Verification items for the finished model (mm, model axes). A direction names the side the tool comes from. Give positions to 0.01 mm unless a question says otherwise; leave off trailing zeros. Write each loop counter-clockwise with the first axis right and the second up, starting at its lowest first coordinate (ties: lowest second). Pieces come first, ordered by that corner, then holes. Notation, with made-up numbers: (47.25, -13.5) - (97.25, -13.5) arc R6 cw to (97.25, -7.5) - close; hole circle Ø3 at (-25.75, 25.5). An arc over 180 degrees is marked (long way). Put each result on its own line as item: value.
from build123d import *

# Parameters (mm, degrees)
BOSS_EXTRUDE1_DEPTH      = 16.65
BOSS_EXTRUDE1_DEPTH_BACK = 16.65
CHAMFER1_SIZE            = 1.5
SKETCH2_R                = 1.75
BOSS_EXTRUDE2_DEPTH      = 1
SKETCH3_R                = 0.6
BOSS_EXTRUDE3_DEPTH      = 5
SKETCH4_W                = 29.3
SKETCH4_H                = 9.15
CUT_EXTRUDE1_DEPTH       = 5.5
CHAMFER2_SIZE            = 0.5


with BuildPart() as part:
    # Sketch1 → Boss-Extrude1 (new, two sides: drawn at the far end of the back side and taken through both)
    with BuildSketch(Plane(origin=(0, 0, 0), x_dir=(0, 0, -1), z_dir=(1, 0, 0)).offset(-BOSS_EXTRUDE1_DEPTH_BACK)):
        Polygon((-24.775, 15.2), (-8.275, 15.2), (-3.825, 10.75), (24.775, 10.75), (24.775, 0), (-16.575, 0), (-19.975, 3.4), (-24.775, 3.4), align=None)
    extrude(amount=BOSS_EXTRUDE1_DEPTH + BOSS_EXTRUDE1_DEPTH_BACK)

    # Chamfer1
    chamfer1_edges = [part.edges().sort_by_distance(p)[0] for p in [
        (-16.65, 1.7, 18.275),
        (-16.65, 0, -4.1),
        (0, 10.75, -24.775),
        (0, 0, -24.775),
        (-16.65, 5.375, -24.775),
        (-16.65, 10.75, -10.475),
        (-16.65, 12.975, 6.05),
        (16.65, 3.4, 22.375),
        (16.65, 1.7, 18.275),
        (16.65, 0, -4.1),
        (16.65, 5.375, -24.775),
        (16.65, 10.75, -10.475),
        (16.65, 12.975, 6.05),
        (16.65, 15.2, 16.525),
        (-16.65, 15.2, 16.525),
        (-16.65, 3.4, 22.375),
    ]]
    chamfer(chamfer1_edges, length=CHAMFER1_SIZE)

    # Sketch2 → Boss-Extrude2 (add)
    with BuildSketch(Plane(origin=(0, 0, -24.775), x_dir=(-1, 0, 0), z_dir=(0, 0, -1))):
        with Locations((-9.45, 6)):
            Circle(SKETCH2_R)
        with Locations((9.55, 6)):
            Circle(SKETCH2_R)
    extrude(amount=BOSS_EXTRUDE2_DEPTH)

    # Sketch3 → Boss-Extrude3 (add)
    with BuildSketch(Plane(origin=(0, 0, -25.775), x_dir=(-1, 0, 0), z_dir=(0, 0, -1))):
        with Locations((-9.45, 6)):
            Circle(SKETCH3_R)
        with Locations((9.55, 6)):
            Circle(SKETCH3_R)
    extrude(amount=BOSS_EXTRUDE3_DEPTH)

    # Sketch4 → Cut-Extrude1 (cut)
    with BuildSketch(Plane.XY.offset(24.775)):
        with Locations((0, 9.3)):
            Rectangle(SKETCH4_W, SKETCH4_H)
    extrude(amount=-CUT_EXTRUDE1_DEPTH, mode=Mode.SUBTRACT)

    # Chamfer2
    chamfer2_edges = [part.edges().sort_by_distance(p)[0] for p in [
        (-14.65, 9.3, 24.775),
        (0, 4.725, 24.775),
        (14.65, 9.3, 24.775),
        (0, 13.875, 24.775),
    ]]
    chamfer(chamfer2_edges, length=CHAMFER2_SIZE)


solid = part.part
Q1. Set-up check for faces 1 (the face through (0, 10.75, -10)), 2 (the face through (0, 13.875, 22)), 3 (the face through (0, 3.4, 22)), 4 (the face through (-9.17, 4.29, -25.27)): record each of +Z, -Z, +X, -X, +Y, -Y from which the full face is reachable in a straight line by a thin tool's end or side.
Answers follow:
face 1: -Z, +X, -X, +Y
face 2: +Z
face 3: +Z, +X, -X, -Y
face 4: -Z
Q2. Go/stop test with flat-tipped pins: pin 1 Ø2.5 at (x, y) = (-6, 3.5) entering from -Z (3 decimals); pin 2 Ø3 at (x, y) = (9, 5.5) entering from -Z (3 decimals); pin 3 Ø6 at (x, y) = (-12, 10) entering from -Z (3 decimals); pin 4 Ø1.5 at (x, z) = (7, 21) entering from -Y. Record where each tip stops, or that it passes through.
Answers follow:
pin 1: stops at z = -24.775
pin 2: stops at z = -30.775
pin 3: stops at z = -25.775
pin 4: stops at y = 3.4
Q3. Section check D-D, the plane x = 14. Record the cut outline in (y, z) (3 decimals), plus the area to 3 significant figures.
Answers follow:
outline: (0, -23.275) - (1.5, -24.775) - (9.25, -24.775) - (10.75, -23.275) - (10.75, 3.825) - (15.2, 8.275) - (15.2, 24.775) - (14.375, 24.775) - (13.875, 24.275) - (13.875, 19.275) - (4.725, 19.275) - (4.725, 24.275) - (4.225, 24.775) - (3.4, 24.775) - (3.4, 19.975) - (0, 16.575) - close
area: 541 mm2
Q4. Section check B-B, the plane y = 6. Record the cut outline in (x, z) (3 decimals), plus the area to 3 significant figures.
Answers follow:
outline: (-16.65, -23.275) - (-15.15, -24.775) - (-11.3, -24.775) - (-11.3, -25.775) - (-10.15, -25.775) - (-10.15, -30.775) - (-8.95, -30.775) - (-8.95, -25.775) - (-7.8, -25.775) - (-7.8, -24.775) - (7.7, -24.775) - (7.7, -25.775) - (8.85, -25.775) - (8.85, -30.775) - (10.05, -30.775) - (10.05, -25.775) - (11.2, -25.775) - (11.2, -24.775) - (15.15, -24.775) - (16.65, -23.275) - (16.65, 24.775) - (15.15, 24.775) - (14.65, 24.275) - (14.65, 19.275) - (-14.65, 19.275) - (-14.65, 24.275) - (-15.15, 24.775) - (-16.65, 24.775) - close
area: 1,510 mm2
Q5. Section check C-C, the plane z = -21. Record the cut outline in (x, y), plus the area to 3 significant figures.
Answers follow:
outline: (-16.65, 1.5) - (-15.15, 0) - (15.15, 0) - (16.65, 1.5) - (16.65, 9.25) - (15.15, 10.75) - (-15.15, 10.75) - (-16.65, 9.25) - close
area: 353 mm2
Q6. Section check A-A, the plane x = -9.55. Record the cut outline in (y, z) (3 decimals), plus the area to 3 significant figures.
Answers follow:
outline: (0, -23.275) - (1.5, -24.775) - (4.25, -24.775) - (4.25, -25.775) - (5.4, -25.775) - (5.4, -30.775) - (6.6, -30.775) - (6.6, -25.775) - (7.75, -25.775) - (7.75, -24.775) - (9.25, -24.775) - (10.75, -23.275) - (10.75, 3.825) - (15.2, 8.275) - (15.2, 24.775) - (14.375, 24.775) - (13.875, 24.275) - (13.875, 19.275) - (4.725, 19.275) - (4.725, 24.275) - (4.225, 24.775) - (3.4, 24.775) - (3.4, 19.975) - (0, 16.575) - close
area: 551 mm2
Q7. Scan lines: line 1 along X through (y, z) = (7.5, 22.5); line 2 along Z through (x, y) = (3, 5.5) (3 decimals); line 3 along Z through (x, y) = (9, 7) (3 decimals). Record each from-to range of solid material in increasing order.
Answers follow:
line 1: x = -16.65 to -14.65, 14.65 to 16.65
line 2: z = -24.775 to 19.275
line 3: z = -25.775 to 19.275
Q8. Release check for a two-part mould opening along X. For faces 5 (the face through (-10, 5, -25.775)), 6 (the face through (-0.212, 0.739, -24.014)), 7 (the face through (15.9, 10, -9.2)) record: released by +X, released by -X, zero draft, split by the parting line, or undercut.
Answers follow:
face 5: undercut
face 6: zero draft
face 7: released by +X
